from build123d import *
from build123d.topology import SkipClean

# Parameters (mm, degrees)
SKETCH1_W            = 106
SKETCH1_H            = 106
BOSS_EXTRUDE1_DEPTH  = 8.5
SHELL1_T             = -2
BOSS_EXTRUDE2_START  = -2
SKETCH2_W            = 15
SKETCH2_H            = 15
BOSS_EXTRUDE2_DEPTH  = 8.5
M5_CLEARANCE_HOLE1_D = 5.8
SKETCH5_R            = 2.9
SKETCH5_W            = 102
SKETCH5_H            = 102
BOSS_EXTRUDE3_DEPTH  = 1.5
FILLET2_R            = 3
SKETCH6_W            = 102
SKETCH6_H            = 102
BOSS_EXTRUDE4_DEPTH  = 0.5


with BuildPart() as part:
    # Sketch1 → Boss-Extrude1 (new body)
    with BuildSketch(Plane(origin=(0, 0, 0), x_dir=(1, 0, 0), z_dir=(0, 1, 0))):
        Rectangle(SKETCH1_W, SKETCH1_H)
    extrude(amount=-BOSS_EXTRUDE1_DEPTH)

    # Shell1
    shell1_openings = [part.faces().sort_by_distance(p)[0] for p in [
        (0, 0, 0),
    ]]
    offset(amount=SHELL1_T, openings=shell1_openings, kind=Kind.INTERSECTION)

    # Sketch2 → Boss-Extrude2 (add)
    with BuildSketch(Plane(origin=(0, -6.5, 0), x_dir=(1, 0, 0), z_dir=(0, 1, 0)).offset(BOSS_EXTRUDE2_START)):
        with Locations((-45.5, 60.5)):
            Rectangle(SKETCH2_W, SKETCH2_H)
        with Locations((45.5, 60.5)):
            Rectangle(SKETCH2_W, SKETCH2_H)
        with Locations((45.5, -60.5)):
            Rectangle(SKETCH2_W, SKETCH2_H)
        with Locations((-45.5, -60.5)):
            Rectangle(SKETCH2_W, SKETCH2_H)
    extrude(amount=BOSS_EXTRUDE2_DEPTH)

    # M5 Clearance Hole1 (through all)
    with Locations(Plane(origin=(0, 0, 0), x_dir=(1, 0, 0), z_dir=(0, 1, 0))):
        with Locations((-45.5, -60.5), (-45.5, 60.5), (45.5, 60.5), (45.5, -60.5)):
            Hole(M5_CLEARANCE_HOLE1_D / 2)

    # Sketch5 → Boss-Extrude3 (add)
    with BuildSketch(Plane(origin=(0, 0, 0), x_dir=(1, 0, 0), z_dir=(0, 1, 0))):
        Polygon((53, -68), (53, 68), (38, 68), (38, 53), (-38, 53), (-38, 68), (-53, 68), (-53, -68), (-38, -68), (-38, -53), (38, -53), (38, -68), align=None)
        with Locations(Location((45.5, -60.5, 0), (0, 0, 270))):
            Circle(SKETCH5_R, mode=Mode.SUBTRACT)
        with Locations(Location((45.5, 60.5, 0), (0, 0, 270))):
            Circle(SKETCH5_R, mode=Mode.SUBTRACT)
        with Locations(Location((-45.5, 60.5, 0), (0, 0, 270))):
            Circle(SKETCH5_R, mode=Mode.SUBTRACT)
        with Locations(Location((-45.5, -60.5, 0), (0, 0, 270))):
            Circle(SKETCH5_R, mode=Mode.SUBTRACT)
        Rectangle(SKETCH5_W, SKETCH5_H, mode=Mode.SUBTRACT)
    extrude(amount=BOSS_EXTRUDE3_DEPTH)

    # Fillet2
    fillet2_edges = [part.edges().sort_by_distance(p)[0] for p in [
        (-53, -3.5, 68),
        (-38, -3.5, 53),
        (-38, -3.5, 68),
        (38, -3.5, 53),
        (53, -3.5, 68),
        (38, -3.5, 68),
        (53, -3.5, -68),
        (38, -3.5, -53),
        (38, -3.5, -68),
        (-53, -3.5, -68),
        (-38, -3.5, -68),
        (-38, -3.5, -53),
    ]]
    fillet(fillet2_edges, radius=FILLET2_R)

    # Sketch6 → Boss-Extrude4 (add)
    with SkipClean():  # the faces are left unmerged after this step: merging them gives an invalid solid
        with BuildSketch(Plane(origin=(0, -6.5, 0), x_dir=(1, 0, 0), z_dir=(0, 1, 0))):
            Rectangle(SKETCH6_W, SKETCH6_H)
        extrude(amount=BOSS_EXTRUDE4_DEPTH)


solid = part.part
Read the model definition and answer for the solid it produces. Units are mm, in the model's axes. A direction names the side the tool comes from. Round coordinates to 2 decimals unless told otherwise and drop trailing zeros. Loops run counter-clockwise (first coordinate to the right, second up) from the corner with the lowest first, then second, coordinate; pieces in that order, holes last. Notation, with made-up numbers: (80.5, 29) - (113.5, 29) arc R11 ccw to (113.5, 37) - close; hole circle Ø11 at (17.25, -5.5). An arc over 180 degrees is marked (long way). One line per question, with ' | ' between items. Start each with the question number.
Q1. Flat-ended cylindrical pins translate along their axes: pin 1 (7.5 mm diameter, centred on x = -45.5, z = 60.5, fed in from -Y); pin 2 (3.5 mm diameter, centred on x = 45.5, z = 60.5, fed in from +Y); pin 3 (2 mm diameter, centred on x = 21.5, y = -5, fed in from -Z); pin 4 (4 mm diameter, centred on x = 19.5, y = 0, fed in from +Z). Find the tip coordinate at first contact, or state that the pin passes through.
Q2. For faces 1 (the flat face through (0, -4, 53)), 2 (the flat face through (-51, -2, 1)), 3 (the flat face through (46, -4, -68)), 4 (the flat face through (-1, -8.5, -1)), 5 (the cylindrical face through (38.86, -3.43, -67.1)), determine the directions among +Z, -Z, +X, -X, +Y, -Y from which every point of the face is accessible in a straight line to the end or side of a thin tool.
Q3. Find the intervals of material crossed by L1, parallel to Z at x = 45.5, y = -4.75; L2, parallel to X at y = -4, z = -60.5; L3, parallel to X at y = -3, z = 20.5, in increasing order.
Q4. Section D-D on z = -15.5 is taken. Give the vertices of the cut face in (x, y).
Q5. Section C-C on y = -4 is taken. Count the separate pieces of the cut face and the enclosed holes in it, plus the area to 3 significant figures.
Q6. Section A-A on x = 45.5 is taken. Give the vertices of the cut face in (y, z), plus the area to 3 significant figures.
Q7. Section B-B on z = 60.5 is taken. Give the vertices of the cut face in (x, y), plus the area to 3 significant figures.
Q8. For a pull along Z with two mould halves and no side action, classify faces 6 (the cylindrical face through (52.14, -3.43, -67.1)), 7 (the cylindrical face through (-37.1, -3.57, 53.86)), 8 (the flat face through (-1, -6, -1)) as +Z half, -Z half, draft (parallel to the pull), parting line (faces both ways), or undercut.
Established:
1) pin 1: y = -8.5 | pin 2: through | pin 3: z = -53 | pin 4: z = 53
2) face 1: +Z, +Y, -Y | face 2: +Y | face 3: -Z, +X, -X, +Y, -Y | face 4: +Z, -Z, +X, -X, -Y | face 5: -Z, +Y, -Y
3) L1: -68 to -63.4, -57.6 to -51, 51 to 57.6, 63.4 to 68 | L2: -53 to -48.4, -42.6 to -38, 38 to 42.6, 48.4 to 53 | L3: -53 to -51, 51 to 53
4) outline: (-53, -8.5) - (53, -8.5) - (53, 1.5) - (51, 1.5) - (51, -6) - (-51, -6) - (-51, 1.5) - (-53, 1.5) - close
5) separate pieces: 1 | enclosed holes: 5 | area: 1,620 mm²
6) outline: (-8.5, -68) - (1.5, -68) - (1.5, -63.4) - (-8.5, -63.4) - close; (-8.5, -57.6) - (1.5, -57.6) - (1.5, -51) - (-6, -51) - (-6, 51) - (1.5, 51) - (1.5, 57.6) - (-8.5, 57.6) - close; (-8.5, 63.4) - (1.5, 63.4) - (1.5, 68) - (-8.5, 68) - close | area: 479 mm²
7) outline: (-53, -8.5) - (-48.4, -8.5) - (-48.4, 1.5) - (-53, 1.5) - close; (-42.6, -8.5) - (-38, -8.5) - (-38, 1.5) - (-42.6, 1.5) - close; (38, -8.5) - (42.6, -8.5) - (42.6, 1.5) - (38, 1.5) - close; (48.4, -8.5) - (53, -8.5) - (53, 1.5) - (48.4, 1.5) - close | area: 184 mm²
8) face 6: -Z half | face 7: +Z half | face 8: undercut
